Build history of the part. All positions in model axes, mm. A direction names the side the tool comes from. Coordinates: 2 decimals unless noted, no trailing zeros.
(1) Two-plate mould, pull along X, no slides. Class faces 1 (the face through (-12, -24, 178)), 2 (the face through (15, 0, 178)), 3 (the face through (-13.479, -7.302, 314.243)): pulls with the +X half, pulls with the -X half, needs draft (parallel to the pull), parting line crosses it, or undercut.
(2) Tool access for faces 4 (the face through (-13.521, 0.44, 133.875)), 5 (the face through (11.6, 27, 144.9)), 6 (the face through (-13.48, -2.3, 57.48)): list every direction of +Z, -Z, +X, -X, +Y, -Y with a clear straight run to the whole face (end or side of a thin tool).
(3) Wall check: L1, parallel to Z at x = 0, y = -28.35; L2, parallel to Y at x = 13.8, z = 373.5; L3, parallel to Y at x = -1.25, z = 3. Give the ranges that are in metal, low to high.
(4) Flat gauge pin, fed straight in: P1, Ø5, axis at y = -12.7, z = 8.003, coming from the -X side. Where does the tip first touch, or does it go through?
Autodesk Inventor part; units mm, degrees
ref_plane "YZ Plane" through (0, 0, 0) normal (1, 0, 0) x (0, 1, 0)
ref_plane "XZ Plane" through (0, 0, 0) normal (0, 1, 0) x (-1, 0, 0)
ref_plane "XY Plane" through (0, 0, 0) normal (0, 0, 1) x (1, 0, 0)
sketch "Sketch1" plane through (0, 0, 0) normal (0, 0, 1) x (1, 0, 0)
  line L0 (-15, -30) -> (15, -30)
  line L1 (15, -30) -> (15, 30)
  line L2 (15, 30) -> (-15, 30)
  line L3 (-15, 30) -> (-15, -30)
  line L4 (-15, -30) -> (15, 30) construction
  line L5 (15, -30) -> (-15, 30) construction
  line L6 (-12, -27) -> (12, -27)
  line L7 (12, -27) -> (12, 27)
  line L8 (12, 27) -> (-12, 27)
  line L9 (-12, 27) -> (-12, -27)
  line L10 (-12, -27) -> (12, 27) construction
  line L11 (12, -27) -> (-12, 27) construction
  point P0 (0, 0)
  dimension "d0" = 30
  dimension "d1" = 60
  dimension "d2" = 24
  dimension "d3" = 54
extrude "Extrusion1" add sketch "Sketch1" along normal blind 385
sketch "Sketch2" plane through (15, -30, 0) normal (1, 0, 0) x (0, 0, -1)
  circle A0 centre (-63.02, 30) radius 6
  line L0 (0, 60) -> (-385, 60)
  line L1 (0, 0) -> (0, 60)
  circle A1 centre (-304.72, 30) radius 12
  circle A2 centre (-183.87, 30) radius 2.75
  line L2 (0, 0) -> (-385, 0)
  circle A3 centre (-123.445, 30) radius 2.75
  circle A4 centre (-244.295, 30) radius 2.75
  circle A5 centre (-373.5, 50) radius 2.1
  circle A6 centre (-373.5, 10) radius 2.1
  line L3 (-385, 60) -> (-385, 0)
  line L4 (-213.87, 30) -> (-153.87, 30) construction
  line L5 (-213.87, 10) -> (-153.87, 10)
  line L6 (-153.87, 50) -> (-213.87, 50)
  arc A7 (-213.87, 50) -> (-213.87, 10) centre (-213.87, 30) ccw
  arc A8 (-153.87, 10) -> (-153.87, 50) centre (-153.87, 30) ccw
  circle A9 centre (-354.72, 30) radius 2.75
  point P0 (0, 30)
  point P1 (-183.87, 30)
  dimension "d6" = 12
  dimension "d7" = 30
  dimension "PulleyHole" = 63.02
  dimension "d18" = 24
  dimension "d19" = 30
  dimension "d20" = 241.7
  dimension "d30" = 5.5
  dimension "d31" = 30
  dimension "d32" = 120.85
  dimension "d33" = 5.5
  dimension "d34" = 5.5
  dimension "d35" = 30
  dimension "d36" = 30
  dimension "d37" = 60.425
  dimension "d38" = 60.425
  dimension "d39" = 4.2
  dimension "d40" = 4.2
  dimension "d41" = 10
  dimension "d42" = 11.5
  dimension "d43" = 10
  dimension "d44" = 11.5
  dimension "d56" = 40
  dimension "d57" = 30.425
  dimension "d59" = 60
  dimension "d60" = 10
  dimension "d82" = 5.5
  dimension "d83" = 110.425
  dimension "d84" = 30
extrude "Extrusion2" cut sketch "Sketch2" against normal blind 30 contours A0 | A1 | A2 | A3 | A4 | A5 | A6 | A9
sketch "Sketch4" plane through (-15, 30, 0) normal (0, 1, 0) x (1, 0, 0)
  circle A0 centre (15, -63.02) radius 7.5 construction
  line L0 (0, 0) -> (0, -385)
  line L1 (30, 0) -> (0, 0)
  line L2 (26, -259.72) -> (4, -259.72)
  line L3 (4, -259.72) -> (4, -349.72)
  line L4 (4, -349.72) -> (26, -349.72)
  line L5 (26, -349.72) -> (26, -259.72)
  line L6 (26, -259.72) -> (4, -349.72) construction
  line L7 (4, -259.72) -> (26, -349.72) construction
  line L8 (4, -259.72) -> (26, -259.72)
  line L9 (26, -259.72) -> (26, -39.72)
  line L10 (26, -39.72) -> (4, -39.72)
  line L11 (4, -39.72) -> (4, -259.72)
  point P0 (15, 0)
  point P1 (15, -304.72)
  dimension "d13" = 15
  dimension "d14" = 15
  dimension "d15" = 63.02
  dimension "d23" = 22
  dimension "d24" = 15
  dimension "d25" = 90
  dimension "d26" = 241.7
  dimension "d28" = 22
  dimension "d29" = 220
extrude "Extrusion4" cut sketch "Sketch4" against normal blind 87.25
sketch "Sketch5" plane through (-15, -30, 0) normal (-1, 0, 0) x (0, 0, 1)
  arc A0 (96.02, 56) -> (88.02, 60) centre (88.02, 50) ccw
  line L0 (88.02, 60) -> (30, 60)
  arc A1 (30, 60) -> (30, 0) centre (30, 30) ccw
  line L1 (30, 0) -> (63.02, 0)
  arc A2 (63.02, 0) -> (78.02, 4.0192) centre (63.02, 30) ccw
  line L2 (78.02, 4.0192) -> (108.02, 21.3397)
  arc A3 (108.02, 21.3397) -> (111.02, 36) centre (103.02, 30) ccw
  line L3 (111.02, 36) -> (96.02, 56)
  circle A4 centre (30, 30) radius 9.75
  circle A5 centre (63.02, 30) radius 9.5
  circle A6 centre (88.02, 55) radius 2.2
  circle A7 centre (30, 4.6) radius 2.2
  circle A8 centre (8.003, 17.3) radius 2.2
  circle A9 centre (8.003, 42.7) radius 2.2
  circle A10 centre (30, 55.4) radius 2.2
  circle A11 centre (103.02, 30) radius 2.75
  point P0 (0, 30)
extrude "Extrusion5" cut sketch "Sketch5" against normal blind 30 contours A8 | A9 | A11
fillet "Fillet1" radius 5 8 edges at (-11, -28.5, 349.72) (11, 28.5, 349.72) (11, -28.5, 349.72) (-11, 28.5, 349.72) (11, 28.5, 39.72) (11, -28.5, 39.72) (-11, 28.5, 39.72) (-11, -28.5, 39.72)
sketch "Sketch6" plane through (0, 0, 0) normal (0, 0, -1) x (-1, 0, 0)
  line L0 (12, 27) -> (12, -27)
  line L1 (12, -27) -> (-12, -27)
  line L2 (-12, -27) -> (-12, 27)
  line L3 (-12, 27) -> (12, 27)
  line L4 (15, -30) -> (-15, -30)
  line L5 (15, 30) -> (15, -30)
  line L6 (-15, 30) -> (15, 30)
  line L7 (-15, -30) -> (-15, 30)
  point P0 (0, 0)
extrude "Extrusion6" add sketch "Sketch6" along normal blind 35
sketch "Sketch8" plane through (-15, -30, 385) normal (-1, 0, 0) x (0, 0, 1)
  line L0 (-231.13, 30) -> (-171.13, 30) construction
  line L1 (-231.13, 10) -> (-171.13, 10)
  line L2 (-171.13, 50) -> (-231.13, 50)
  arc A0 (-231.13, 50) -> (-231.13, 10) centre (-231.13, 30) ccw
  arc A1 (-171.13, 10) -> (-171.13, 50) centre (-171.13, 30) ccw
  line L3 (-231.13, 30) -> (-171.13, 30) construction
  line L4 (0, 0) -> (-420, 0)
  circle A2 centre (-261.555, 30) radius 2.75
  point P0 (-385, 30)
  point P1 (-201.13, 30)
  dimension "d61" = 60
  dimension "d62" = 0
  dimension "d63" = 40
  dimension "d64" = 10
  dimension "d65" = 30.425
extrude "Extrusion8" cut sketch "Sketch8" against normal blind 10 contours A0 L2 A1 L1
sketch "Sketch9" plane through (-15, 30, 385) normal (0, 1, 0) x (1, 0, 0)
  circle A0 centre (15, 413) radius 2.75
  circle A1 centre (15, 397) radius 2.75
  line L0 (0, 420) -> (0, 0)
  line L1 (0, 420) -> (30, 420)
  circle A2 centre (15, 7) radius 2.75
  circle A3 centre (15, 23) radius 2.75
  line L2 (30, 0) -> (0, 0)
  point P0 (15, 385)
  dimension "d68" = 5.5
  dimension "d69" = 5.5
  dimension "d70" = 15
  dimension "d71" = 15
  dimension "d72" = 7
  dimension "d73" = 16
  dimension "d74" = 5.5
  dimension "d75" = 5.5
  dimension "d76" = 15
  dimension "d77" = 15
  dimension "d78" = 7
  dimension "d79" = 16
extrude "Extrusion9" cut sketch "Sketch9" against normal up to surface (60 mm away)
equation "\"d15\" = PulleyHole"
properties part number "SideExtrusion" material "Aluminum 6061"
Response values:
1. face 1: undercut
1. face 2: pulls with the +X half
1. face 3: needs draft
2. face 4: -X
2. face 5: +Z, -Z
2. face 6: +X, -X
3. L1: z = -35 to -30.75, -25.25 to -14.75, -9.25 to 39.72, 349.72 to 359.25, 364.75 to 375.25, 380.75 to 385
3. L2: y = -30 to -22.1, -17.9 to 17.9, 22.1 to 30
3. L3: y = -30 to -27, 27 to 30
4. P1: stops at x = -15
